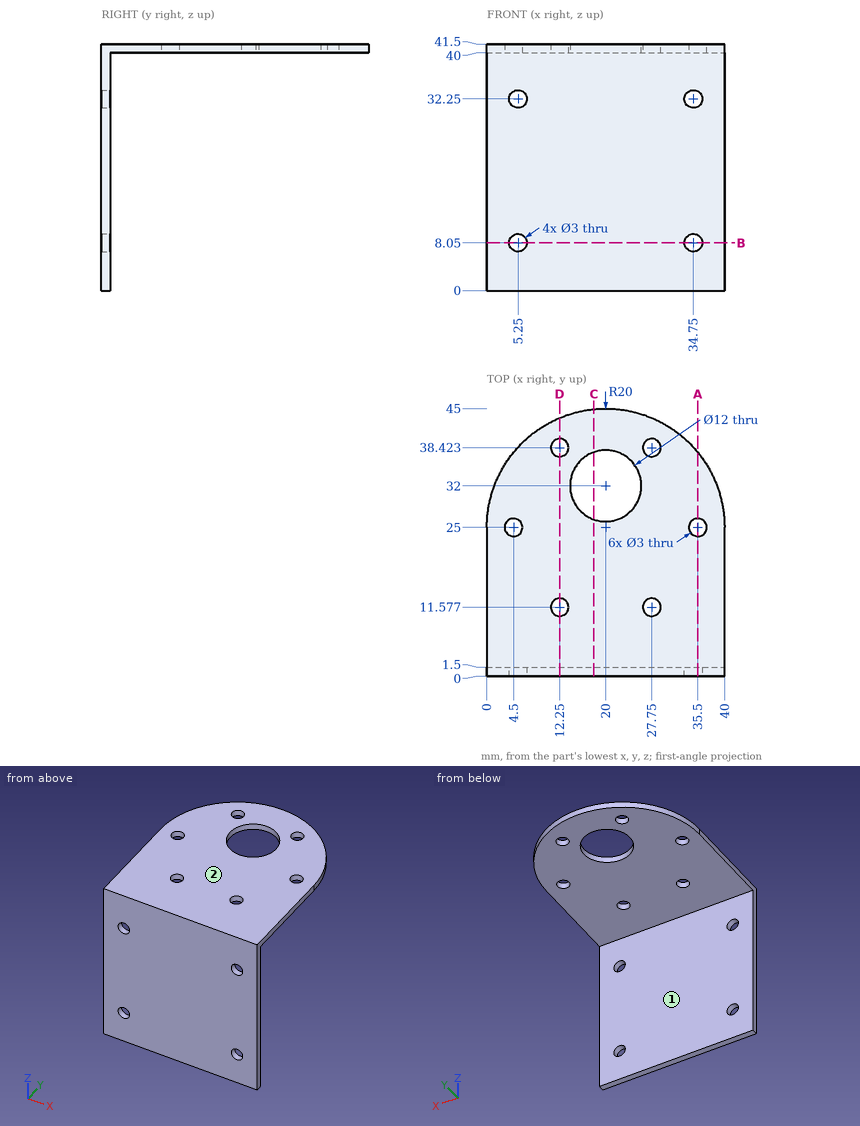
Geometry: see drawing. Coordinates: mm, zero at the bounding-box minimum. A direction names the side the tool comes from. Give positions to 0.01 mm unless a question says otherwise; leave off trailing zeros. Write each loop counter-clockwise with the first axis right and the second up, starting at its lowest first coordinate (ties: lowest second). Pieces come first, ordered by that corner, then holes. Notation, with made-up numbers: (4, 84) -> (60, 84) arc R16 ccw to (60, 111) -> close; hole circle Ø3 at (-15, 50). An arc over 180 degrees is marked (long way). Use one line per item in the form item = value. Start each with the question number.
1) Section query D-D on x = 12.25. Return the cut outline in (y, z), then the cut area to 3 significant figures.
2) Pin query (flat end, axial travel): pin 1 (1.8 mm diameter, centred on x = 5.25, z = 8.05, fed in from +Y); pin 2 (4 mm diameter, centred on x = 12.25, y = 38.42, fed in from -Z); pin 3 (20 mm diameter, centred on x = 14, z = 26, fed in from +Y). Return the tip coordinate at first contact, or that it passes through.
3) Section query A-A on x = 35.5. Return the cut outline in (y, z), then the cut area to 3 significant figures.
4) Section query B-B on z = 8.05. Return the cut outline in (x, y).
5) Ray query, probe 1 along Z at (x, y) = (34.75, 1.15); probe 2 along X at (y, z) = (0.7, 8.05); probe 3 along Y at (x, z) = (27.75, 41). Return the intervals inside material, ascending. Write a range as from..to.
6) Section query C-C on x = 18. Return the cut outline in (y, z).
7) Set-up query: the marked faces 1 and 2. Return all of +Z, -Z, +X, -X, +Y, -Y with unobstructed straight access to the full face (end or side cutting, diameter ignored); none if empty.
Outcome:
q1.outline = (0, 0) -> (1.5, 0) -> (1.5, 40) -> (10.08, 40) -> (10.08, 41.5) -> (0, 41.5) -> close; (13.08, 40) -> (36.92, 40) -> (36.92, 41.5) -> (13.08, 41.5) -> close; (39.92, 40) -> (43.44, 40) -> (43.44, 41.5) -> (39.92, 41.5) -> close
q1.area = 116 mm^2
q2.pin_1 = through
q2.pin_2 = 40
q2.pin_3 = 1.5
q3.outline = (0, 0) -> (1.5, 0) -> (1.5, 6.75) -> (0, 6.75) -> close; (0, 9.35) -> (1.5, 9.35) -> (1.5, 30.95) -> (0, 30.95) -> close; (0, 33.55) -> (1.5, 33.55) -> (1.5, 40) -> (23.5, 40) -> (23.5, 41.5) -> (0, 41.5) -> close; (26.5, 40) -> (37.64, 40) -> (37.64, 41.5) -> (26.5, 41.5) -> close
q3.area = 104 mm^2
q4.outline = (0, 0) -> (3.75, 0) -> (3.75, 1.5) -> (0, 1.5) -> close; (6.75, 0) -> (33.25, 0) -> (33.25, 1.5) -> (6.75, 1.5) -> close; (36.25, 0) -> (40, 0) -> (40, 1.5) -> (36.25, 1.5) -> close
q5.probe_1 = 0..6.55, 9.55..30.75, 33.75..41.5
q5.probe_2 = 0..3.75, 6.75..33.25, 36.25..40
q5.probe_3 = 0..10.08, 13.08..36.92, 39.92..43.44
q6.outline = (0, 0) -> (1.5, 0) -> (1.5, 40) -> (26.34, 40) -> (26.34, 41.5) -> (0, 41.5) -> close; (37.66, 40) -> (44.9, 40) -> (44.9, 41.5) -> (37.66, 41.5) -> close
q7.face_1 = -Z, +X, -X, +Y
q7.face_2 = +Z, +X, -X, +Y, -Y
